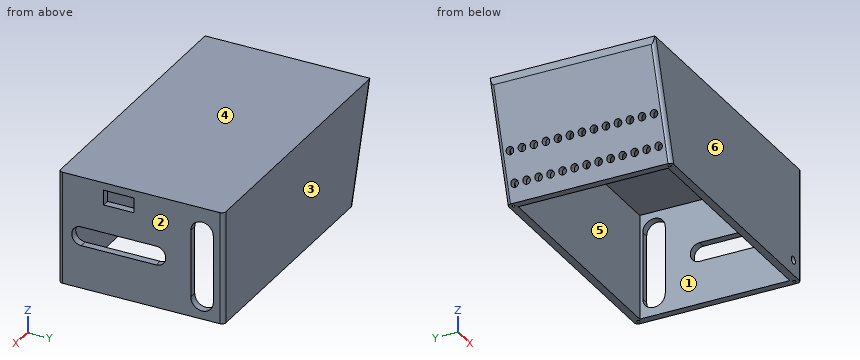
```python
from build123d import *

# Parameters (mm, degrees)
ESQUISSE1_W             = 185
ESQUISSE1_H             = 110
BOSS_EXTRU_1_DEPTH      = 5
BOSS_EXTRU_2_DEPTH      = 110
BOSS_EXTRU_3_DEPTH      = 5
BOSS_EXTRU_4_DEPTH      = 5
ESQUISSE8_W             = 70
ESQUISSE8_H             = 100
BOSS_EXTRU_6_DEPTH      = 5
ESQUISSE10_R            = 2.5
ENL_V_MAT_EXTRU_1_DEPTH = 5
ESQUISSE13_R            = 1
ENL_V_MAT_EXTRU_2_DEPTH = 10
ESQUISSE15_W            = 10
ESQUISSE15_H            = 20
ENL_V_MAT_EXTRU_3_DEPTH = 10
ESQUISSE14_R            = 2.5
ENL_V_MAT_EXTRU_4_DEPTH = 10
CONG_2_R                = 2.5
CONG_3_R                = 2.5
CONG_4_R                = 2.5
CONG_5_R                = 2.5


with BuildPart() as part:
    # Esquisse1 → Boss.-Extru.1 (new body)
    with BuildSketch(Plane.XY):
        with Locations((-22.430690869, -9.25879397)):
            Rectangle(ESQUISSE1_W, ESQUISSE1_H)
    extrude(amount=BOSS_EXTRU_1_DEPTH)

    # Esquisse3 → Boss.-Extru.2 (add)
    with BuildSketch(Plane(origin=(0, 45.74120603, 0), x_dir=(1, 0, 0), z_dir=(0, 1, 0))):
        Polygon((-114.930690869, 0), (-93.616299119, 70), (-88.616299119, 70), (-109.930690869, 0), align=None)
    extrude(amount=-BOSS_EXTRU_2_DEPTH)

    # Esquisse4 → Boss.-Extru.3 (add)
    with BuildSketch(Plane(origin=(0, 45.74120603, 0), x_dir=(1, 0, 0), z_dir=(0, 1, 0))):
        Polygon((-109.930690869, 0), (-88.616299119, 70), (70.069309131, 70), (70.069309131, 0), align=None)
    extrude(amount=-BOSS_EXTRU_3_DEPTH)

    # Esquisse7 → Boss.-Extru.4 (add)
    with BuildSketch(Plane.XZ.offset(64.25879397)):
        Polygon((-109.930690869, 0), (-88.616299119, -70), (70.069309131, -70), (70.069309131, 0), align=None)
    extrude(amount=-BOSS_EXTRU_4_DEPTH)

    # Esquisse8 → Boss.-Extru.6 (add)
    with BuildSketch(Plane(origin=(70.069309131, 0, 0), x_dir=(0, 0, -1), z_dir=(1, 0, 0))):
        with Locations((35, -9.25879397)):
            Rectangle(ESQUISSE8_W, ESQUISSE8_H)
        with BuildLine():
            Line((41.331742872, 0.74120603), (41.331742872, -49.25879397))
            ThreePointArc((41.331742872, -49.25879397), (35, -55.590536842), (28.668257128, -49.25879397))
            Line((28.668257128, -49.25879397), (28.668257128, 0.74120603))
            ThreePointArc((28.668257128, 0.74120603), (35, 7.072948902), (41.331742872, 0.74120603))
        make_face(mode=Mode.SUBTRACT)
        with BuildLine():
            Line((12, 38.74120603), (57, 38.74120603))
            ThreePointArc((57, 38.74120603), (64.5, 31.24120603), (57, 23.74120603))
            Line((57, 23.74120603), (12, 23.74120603))
            ThreePointArc((12, 23.74120603), (4.5, 31.24120603), (12, 38.74120603))
        make_face(mode=Mode.SUBTRACT)
    extrude(amount=-BOSS_EXTRU_6_DEPTH)

    # Esquisse10 → Enlèv. mat.-Extru.1 (cut)
    with BuildSketch(Plane(origin=(-105.179022211, 0, -32.026098333), x_dir=(-0.291287239, 0, 0.956635638), z_dir=(-0.956635638, 0, -0.291287239))):
        with Locations((-8, 38.74120603)):
            Circle(ESQUISSE10_R)
        with Locations((-8, 30.74120603)):
            Circle(ESQUISSE10_R)
        with Locations((-8, 22.74120603)):
            Circle(ESQUISSE10_R)
        with Locations((-8, 14.74120603)):
            Circle(ESQUISSE10_R)
        with Locations((-8, 6.74120603)):
            Circle(ESQUISSE10_R)
        with Locations((-8, -1.25879397)):
            Circle(ESQUISSE10_R)
        with Locations((-8, -9.25879397)):
            Circle(ESQUISSE10_R)
        with Locations((-8, -17.25879397)):
            Circle(ESQUISSE10_R)
        with Locations((-8, -25.25879397)):
            Circle(ESQUISSE10_R)
        with Locations((-8, -33.25879397)):
            Circle(ESQUISSE10_R)
        with Locations((-8, -41.25879397)):
            Circle(ESQUISSE10_R)
        with Locations((-8, -49.25879397)):
            Circle(ESQUISSE10_R)
        with Locations((-8, -57.25879397)):
            Circle(ESQUISSE10_R)
        with Locations((-28, -57.25879397)):
            Circle(ESQUISSE10_R)
        with Locations((-28, -49.25879397)):
            Circle(ESQUISSE10_R)
        with Locations((-28, -41.25879397)):
            Circle(ESQUISSE10_R)
        with Locations((-28, -9.25879397)):
            Circle(ESQUISSE10_R)
        with Locations((-28, -17.25879397)):
            Circle(ESQUISSE10_R)
        with Locations((-28, -25.25879397)):
            Circle(ESQUISSE10_R)
        with Locations((-28, -33.25879397)):
            Circle(ESQUISSE10_R)
        with Locations((-28, -1.25879397)):
            Circle(ESQUISSE10_R)
        with Locations((-28, 6.74120603)):
            Circle(ESQUISSE10_R)
        with Locations((-28, 14.74120603)):
            Circle(ESQUISSE10_R)
        with Locations((-28, 22.74120603)):
            Circle(ESQUISSE10_R)
        with Locations((-28, 30.74120603)):
            Circle(ESQUISSE10_R)
        with Locations((-28, 38.74120603)):
            Circle(ESQUISSE10_R)
    extrude(amount=-ENL_V_MAT_EXTRU_1_DEPTH, mode=Mode.SUBTRACT)

    # Esquisse13 → Enlèv. mat.-Extru.2 (cut)
    with BuildSketch(Plane(origin=(0, 0, -70), x_dir=(-1, 0, 0), z_dir=(0, 0, -1))):
        with Locations((-67.069309131, 42.74120603)):
            Circle(ESQUISSE13_R)
        with Locations((-67.069309131, -61.25879397)):
            Circle(ESQUISSE13_R)
        with Locations((90.616299119, -61.25879397)):
            Circle(ESQUISSE13_R)
        with Locations((90.616299119, 42.74120603)):
            Circle(ESQUISSE13_R)
    extrude(amount=-ENL_V_MAT_EXTRU_2_DEPTH, mode=Mode.SUBTRACT)

    # Esquisse15 → Enlèv. mat.-Extru.3 (cut)
    with BuildSketch(Plane(origin=(70.069309131, 0, 0), x_dir=(0, 0, -1), z_dir=(1, 0, 0))):
        with Locations((5, -24.25879397)):
            Rectangle(ESQUISSE15_W, ESQUISSE15_H)
    extrude(amount=-ENL_V_MAT_EXTRU_3_DEPTH, mode=Mode.SUBTRACT)

    # Esquisse14 → Enlèv. mat.-Extru.4 (cut)
    with BuildSketch(Plane(origin=(0, -64.25879397, 0), x_dir=(-1, 0, 0), z_dir=(0, -1, 0))):
        with Locations((-60.069309131, 60)):
            Circle(ESQUISSE14_R)
    extrude(amount=-ENL_V_MAT_EXTRU_4_DEPTH, mode=Mode.SUBTRACT)

    # Congé2
    cong_2_edges = [part.edges().sort_by_distance(p)[0] for p in [
        (-104.273494994, -64.25879397, -35),
    ]]
    fillet(cong_2_edges, radius=CONG_2_R)

    # Congé3
    cong_3_edges = [part.edges().sort_by_distance(p)[0] for p in [
        (-104.273494994, 45.74120603, -35),
    ]]
    fillet(cong_3_edges, radius=CONG_3_R)

    # Congé4
    cong_4_edges = [part.edges().sort_by_distance(p)[0] for p in [
        (70.069309131, -64.25879397, -32.5),
    ]]
    fillet(cong_4_edges, radius=CONG_4_R)

    # Congé5
    cong_5_edges = [part.edges().sort_by_distance(p)[0] for p in [
        (70.069309131, 45.74120603, -32.5),
    ]]
    fillet(cong_5_edges, radius=CONG_5_R)


solid = part.part
```
Verification items for the finished model (mm, model axes). Face numbers are marked on the shaded views. A direction names the side the tool comes from. Coordinates: 2 decimals unless noted, no trailing zeros. Write each loop counter-clockwise with the first axis right and the second up, starting at its lowest first coordinate (ties: lowest second). Pieces come first, ordered by that corner, then holes. Notation, with made-up numbers: M 29.25,65 L 49.25,65 A8 cw 49.25,75 Z; hole C -10,7 d2. An arc over 180 degrees is marked long. Answer as a JSON object with one key per item and string values. Group by question number.
(1) Cross-section at A-A, the plane x = 17.5. Record the cut outline in (y, z).
(2) Material ranges on line 1 (Y direction, x = 60, z = -45.5); line 2 (Z direction, x = -41.5, y = -17.5); line 3 (X direction, y = -18, z = -14.5), recorded low to high.
(3) Tool access check on the marked faces 1 and 2. Record the directions out of +Z, -Z, +X, -X, +Y, -Y that give a thin tool (end or side, any length) a straight path to the whole face; none if there is none.
(4) Release check for a two-part mould opening along Y. For the marked faces 3, 4, 5 and 6 record: +Y half, -Y half, draft (parallel to the pull), parting line (faces both ways), or undercut.
(5) Gauge pin test, flat ends, axial feed: pin 1 (5 mm diameter, centred on x = -71, y = -27.5, fed in from -Z); pin 2 (0.6 mm diameter, centred on x = 67, y = 42.5, fed in from -Z); pin 3 (1 mm diameter, centred on y = 32, z = -38, fed in from -X). Record the tip position at first contact, or that the pin passes through.
Reply:
{
 "1": {"outline": "M -64.26,-70 L -59.26,-70 L -59.26,0 L 40.74,0 L 40.74,-70 L 45.74,-70 L 45.74,5 L -64.26,5 Z"},
 "2": {"line 1": "-64.26 to -59.26, 40.74 to 45.74", "line 2": "0 to 5", "line 3": "-110.52 to -105.52, 65.07 to 70.07"},
 "3": {"face 1": "-Z", "face 2": "+Z, -Z, +X, +Y, -Y"},
 "4": {"face 3": "+Y half", "face 4": "draft", "face 5": "undercut", "face 6": "-Y half"},
 "5": {"pin 1": "z = 0", "pin 2": "z = -60", "pin 3": "x = -103.51"}
}
